```python
from build123d import *

# Parameters (mm, degrees)
SKETCH_R        = 2
PAD_DEPTH       = 5
SKETCH001_R     = 13
PAD001_DEPTH    = 9
SKETCH002_R     = 8
POCKET_DEPTH    = 18.001
SKETCH003_W     = 37.242641
SKETCH003_H     = 5
POCKET001_DEPTH = 41.926514
SKETCH004_R     = 11.35
POCKET002_DEPTH = 13
CHAMFER_SIZE    = 3.1
SKETCH005_W     = 40
SKETCH005_H     = 4
POCKET003_DEPTH = 41.926514


with BuildPart() as part:
    # Sketch → Pad (new body)
    with BuildSketch(Plane.XY):
        with BuildLine():
            Line((1.414214, 0), (49.84062, 0))
            ThreePointArc((49.84062, 0), (51.688379, 1.234633), (51.254834, 3.414214))
            Line((51.254834, 3.414214), (27.041631, 27.627417))
            ThreePointArc((27.041631, 27.627417), (25.627417, 28.213203), (24.213203, 27.627417))
            Line((0, 3.414214), (24.213203, 27.627417))
            ThreePointArc((0, 3.414214), (-0.433546, 1.234633), (1.414214, 0))
        make_face()
        with Locations((4.414214, 3.25)):
            Circle(SKETCH_R, mode=Mode.SUBTRACT)
        with Locations((46.84062, 3.25)):
            Circle(SKETCH_R, mode=Mode.SUBTRACT)
        with Locations((25.627417, 24.463203)):
            Circle(SKETCH_R, mode=Mode.SUBTRACT)
    extrude(amount=PAD_DEPTH)

    # Sketch001 (on Face10 of Pad) → Pad001 (join, symmetric)
    with BuildSketch(Plane(origin=(0, 0, 0), x_dir=(1, 0, 0), z_dir=(0, 0, -1))):
        with Locations((25.627417, -8.963203)):
            Circle(SKETCH001_R)
    extrude(amount=PAD001_DEPTH, both=True)

    # Sketch002 (on Face15 of Pad001) → Pocket (cut, through all)
    with BuildSketch(Plane(origin=(0, 0, -9), x_dir=(1, 0, 0), z_dir=(0, 0, -1))):
        with Locations((25.627417, -8.963203)):
            Circle(SKETCH002_R)
    extrude(amount=-POCKET_DEPTH, mode=Mode.SUBTRACT)

    # Sketch003 (on Face8 of Pocket) → Pocket001 (cut, through all)
    with BuildSketch(Plane(origin=(27.334524, 27.334524, 0), x_dir=(-0.707107, 0.707107, 0), z_dir=(0.707107, 0.707107, 0))):
        with Locations((-15.207106, 7.5)):
            Rectangle(SKETCH003_W, SKETCH003_H)
    extrude(amount=-POCKET001_DEPTH, mode=Mode.SUBTRACT)

    # Sketch004 (on Face15 of Pocket001) → Pocket002 (cut)
    with BuildSketch(Plane.XY.offset(5)):
        with Locations((25.627417, 8.963203)):
            Circle(SKETCH004_R)
    extrude(amount=-POCKET002_DEPTH, mode=Mode.SUBTRACT)

    # Chamfer
    chamfer_edges = [part.edges().sort_by_distance(p)[0] for p in [
        (14.277417, 8.963203, -8),
    ]]
    chamfer(chamfer_edges, length=CHAMFER_SIZE)

    # Sketch005 (on Face12 of Chamfer) → Pocket003 (cut, through all)
    with BuildSketch(Plane(origin=(-1.707107, 1.707107, 0), x_dir=(-0.707107, -0.707107, 0), z_dir=(-0.707107, 0.707107, 0))):
        with Locations((-20, 5)):
            Rectangle(SKETCH005_W, SKETCH005_H)
    extrude(amount=-POCKET003_DEPTH, mode=Mode.SUBTRACT)


solid = part.part
```
Input: part model. Units: mm. Frame: model coordinates. A direction names the side the tool comes from. Coordinates: 2 decimals unless noted, no trailing zeros. Write each loop counter-clockwise with the first axis right and the second up, starting at its lowest first coordinate (ties: lowest second). Pieces come first, ordered by that corner, then holes.
1) Mould query, pull axis Y, two halves, no side actions, for faces 5 (the flat face through (39.32, 15.35, 1.48)), 6 (the conical face through (33.64, 11.49, -7.85)), 7 (the flat face through (9, 0, 1)). Classes: pulls with the +Y half, pulls with the -Y half, needs draft (parallel to the pull), parting line crosses it, or undercut.
2) Section D-D on x = 10.5. Output: boundary loops of the cut face in (y, z), and give its area (3 significant figures).
3) Section A-A on z = -6.25. Output: boundary loops of the cut face in (x, y).
4) Section B-B on x = 42.5. Output: boundary loops of the cut face in (y, z), and give its area (3 significant figures).
5) Section C-C on z = -1. Output: boundary loops of the cut face in (x, y), and give its area (3 significant figures).
6) Material intervals for line 1 along Y through (x, z) = (24, 2.5); line 2 along X through (y, z) = (8.5, -1.75); line 3 along X through (y, z) = (6, -1.5), sorted ascending.
7) Set-up query: faces 1 (the cylindrical face through (23.935, -3.926, -4.417)), 2 (the cylindrical face through (26.55, 22.69, 1.48)), 3 (the flat face through (42, 0, 1)), 4 (the cylindrical face through (17.26, 16.63, -0.89)). Return all of +Z, -Z, +X, -X, +Y, -Y with unobstructed straight access to the full face (end or side cutting, diameter ignored); none if empty.
8) Pin query (flat end, axial travel): pin 1 Ø18.5 at (x, y) = (25.63, 8.96) entering from +Z; pin 2 Ø6.5 at (x, y) = (4.41, 3.25) entering from -Z; pin 3 Ø0.9 at (x, z) = (40, 1.5) entering from -Y; pin 4 Ø2 at (x, y) = (42, 15) entering from -Z. Return the tip coordinate at first contact, or that it passes through.
Check result:
1. face 5: pulls with the +Y half
1. face 6: undercut
1. face 7: pulls with the -Y half
2. outline: (0, 0) - (13.91, 0) - (13.91, 3) - (0, 3) - close
2. area: 41.7 mm2
3. outline: circle Ø26 at (25.63, 8.96); hole circle Ø20 at (25.63, 8.96)
4. outline: (0, 0) - (12.17, 0) - (12.17, 3) - (0, 3) - close
4. area: 36.5 mm2
5. outline: circle Ø26 at (25.63, 8.96); hole circle Ø22.7 at (25.63, 8.96)
5. area: 126 mm2
6. line 1: y = -3.93 to -2.27, 20.2 to 23.3, 25.63 to 27.41
6. line 2: x = 12.64 to 14.29, 36.97 to 38.62
6. line 3: x = 12.97 to 14.67, 36.58 to 38.29
7. face 1: -Z
7. face 2: +Z, -Z
7. face 3: +Z, -Z, +X, -Y
7. face 4: +Z
8. pin 1: stops at z = -7
8. pin 2: stops at z = 0
8. pin 3: stops at y = 0
8. pin 4: passes through
